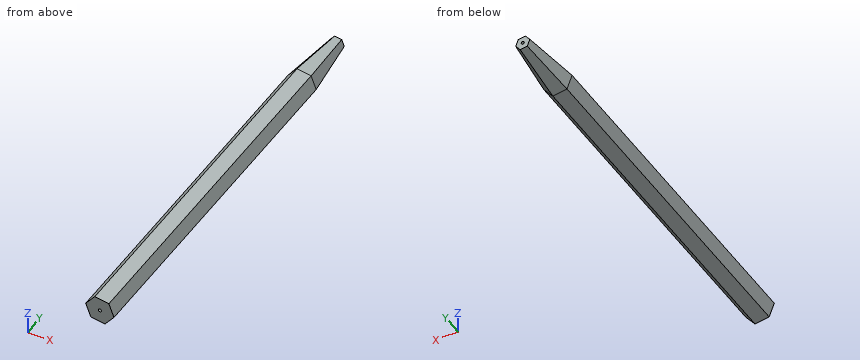
from build123d import *
from OCP.BRepFilletAPI import BRepFilletAPI_MakeChamfer

# Parameters (mm, degrees)
SKIZZE1_R                       = 0.5
AUFSATZ_LINEAR_AUSTRAGEN1_DEPTH = 135
FASE2_SIZE                      = 20
FASE2_SIZE2                     = 2


with BuildPart() as part:
    # Skizze1 → Aufsatz-Linear austragen1 (new body)
    with BuildSketch(Plane(origin=(0, 0, 0), x_dir=(1, 0, 0), z_dir=(0, 1, 0))):
        Polygon((2.912582575, -3.584717015), (4.560747288, 0.730011993), (1.648164713, 4.314729008), (-2.912582575, 3.584717015), (-4.560747288, -0.730011993), (-1.648164713, -4.314729008), align=None)
        with Locations(Location((0, 0, 0), (0, 0, 270))):
            Circle(SKIZZE1_R, mode=Mode.SUBTRACT)
    extrude(amount=AUFSATZ_LINEAR_AUSTRAGEN1_DEPTH)

    # Fase2: one chamfer whose edges measure the first distance from different faces: ONE call of the kernel's chamfer builder (chamfer() names one face for all edges)
    fase2_edges_1 = [part.edges().sort_by_distance(p)[0] for p in [
        (3.104456, 135, -2.5223705),
    ]]
    fase2_side_1 = [part.faces().sort_by_distance(p)[0] for p in [
        (3.104456, 67.5, -2.5223705),
    ]]
    fase2_edges_2 = [part.edges().sort_by_distance(p)[0] for p in [
        (-0.632208931, 135, -3.949723012),
    ]]
    fase2_side_2 = [part.faces().sort_by_distance(p)[0] for p in [
        (-0.632208931, 67.5, -3.949723012),
    ]]
    fase2_edges_3 = [part.edges().sort_by_distance(p)[0] for p in [
        (-3.736664931, 135, -1.427352511),
    ]]
    fase2_side_3 = [part.faces().sort_by_distance(p)[0] for p in [
        (-3.736664931, 67.5, -1.427352511),
    ]]
    fase2_edges_4 = [part.edges().sort_by_distance(p)[0] for p in [
        (-3.104456, 135, 2.5223705),
    ]]
    fase2_side_4 = [part.faces().sort_by_distance(p)[0] for p in [
        (-3.104456, 67.5, 2.5223705),
    ]]
    fase2_edges_5 = [part.edges().sort_by_distance(p)[0] for p in [
        (0.632208931, 135, 3.949723012),
    ]]
    fase2_side_5 = [part.faces().sort_by_distance(p)[0] for p in [
        (0.632208931, 67.5, 3.949723012),
    ]]
    fase2_edges_6 = [part.edges().sort_by_distance(p)[0] for p in [
        (3.736664931, 135, 1.427352511),
    ]]
    fase2_side_6 = [part.faces().sort_by_distance(p)[0] for p in [
        (3.736664931, 67.5, 1.427352511),
    ]]
    fase2 = BRepFilletAPI_MakeChamfer(part.part.solid().wrapped)
    for e in fase2_edges_1:
        fase2.Add(FASE2_SIZE, FASE2_SIZE2, e.wrapped, fase2_side_1[0].wrapped)  # the first distance lies on this face
    for e in fase2_edges_2:
        fase2.Add(FASE2_SIZE, FASE2_SIZE2, e.wrapped, fase2_side_2[0].wrapped)  # the first distance lies on this face
    for e in fase2_edges_3:
        fase2.Add(FASE2_SIZE, FASE2_SIZE2, e.wrapped, fase2_side_3[0].wrapped)  # the first distance lies on this face
    for e in fase2_edges_4:
        fase2.Add(FASE2_SIZE, FASE2_SIZE2, e.wrapped, fase2_side_4[0].wrapped)  # the first distance lies on this face
    for e in fase2_edges_5:
        fase2.Add(FASE2_SIZE, FASE2_SIZE2, e.wrapped, fase2_side_5[0].wrapped)  # the first distance lies on this face
    for e in fase2_edges_6:
        fase2.Add(FASE2_SIZE, FASE2_SIZE2, e.wrapped, fase2_side_6[0].wrapped)  # the first distance lies on this face
    add(Compound.cast(fase2.Shape()), mode=Mode.REPLACE)


solid = part.part
Input: part model. Units: mm. Frame: model coordinates. Give positions to 0.01 mm unless a question says otherwise; leave off trailing zeros. Order: outer loops, then holes, each group sorted by start corner. A loop starts at its lowest first (then second) coordinate and runs counter-clockwise, first axis right, second up. Notation, with made-up numbers: (75, 32) - (114, 32) arc R16 ccw to (114, 60) - close; hole circle Ø9 at (23, 9). An arc over 180 degrees is marked (long way). Answer as a JSON object with one key per item and string values. Group by question number.
Q1. Cut plane B-B, the plane y = 126.5. Output: boundary loops of the cut face in (x, z).
Q2. Line query: probe 1 along X at (y, z) = (82, 0); probe 2 along Z at (x, y) = (-1.25, 116); probe 3 along X at (y, z) = (60, 2.25). Output: solid intervals per line, ascending.
Q3. First-contact query: pin 1 Ø5 at (y, z) = (84.5, -1.5) entering from -X; pin 2 Ø2 at (y, z) = (18, 2.5) entering from +X; pin 3 Ø1.5 at (x, y) = (1, 84.5) entering from +Z. Flat tips, straight axial feed; report the tip coordinate or a pass-through.
Q4. Cut plane A-A, the plane y = 92.5. Output: boundary loops of the cut face in (x, z), then the cut area to 3 significant figures.
Results:
{
 "1": {"outline": "(-3.25, 0.52) - (-2.08, -2.55) - (1.17, -3.07) - (3.25, -0.52) - (2.08, 2.55) - (-1.17, 3.07) - close; hole circle Ø1 at (0, 0)"},
 "2": {"probe 1": "-4.28 to -0.5, 0.5 to 4.28", "probe 2": "-3.75 to 4.15", "probe 3": "-3.33 to 3.42"},
 "3": {"pin 1": "x = -4.56", "pin 2": "x = 3.71", "pin 3": "z = 4.01"},
 "4": {"outline": "(-4.56, 0.73) - (-2.91, -3.58) - (1.65, -4.31) - (4.56, -0.73) - (2.91, 3.58) - (-1.65, 4.31) - close; hole circle Ø1 at (0, 0)", "area": "54.6 mm^2"}
}
